For this review, use the dimensioned drawing (mm, ordinates from the lowest corner) and the shaded views. Give positions to 0.01 mm unless a question says otherwise; leave off trailing zeros. Loops run counter-clockwise (first coordinate to the right, second up) from the corner with the lowest first, then second, coordinate; pieces in that order, holes last. Notation, with made-up numbers: (-38.75, -27) -> (2.25, -27) arc R30 ccw to (2.25, 3) -> close; hole circle Ø4 at (32.5, 14). An arc over 180 degrees is marked (long way). Use a Markdown table: item, result. Add a question column.
1. Add section D-D (z = 43.5). State the section outline as (x, y) points.
2. Add section C-C (x = 2.2). Count the separate pieces of the cut face and the enclosed holes in it, and give its area (3 significant figures).
3. Add section B-B (z = 30). State the section outline as (x, y) points.
4. For pin 1 Ø4 at (y, z) = (79, 47.5) entering from -X, flat-tipped, find the tip position at first contact; note if it passes through.
5. To check wall thickness, follow line 1 (Y direction, x = 2.1, z = 35.5); line 2 (Y direction, x = 2.35, z = 44); line 3 (Z direction, x = 0.8, y = 74.5). State the ranges of each line that lie inside material, in increasing order.
6. Add section A-A (y = 44). State the section outline as (x, z) points, and give its area (3 significant figures).
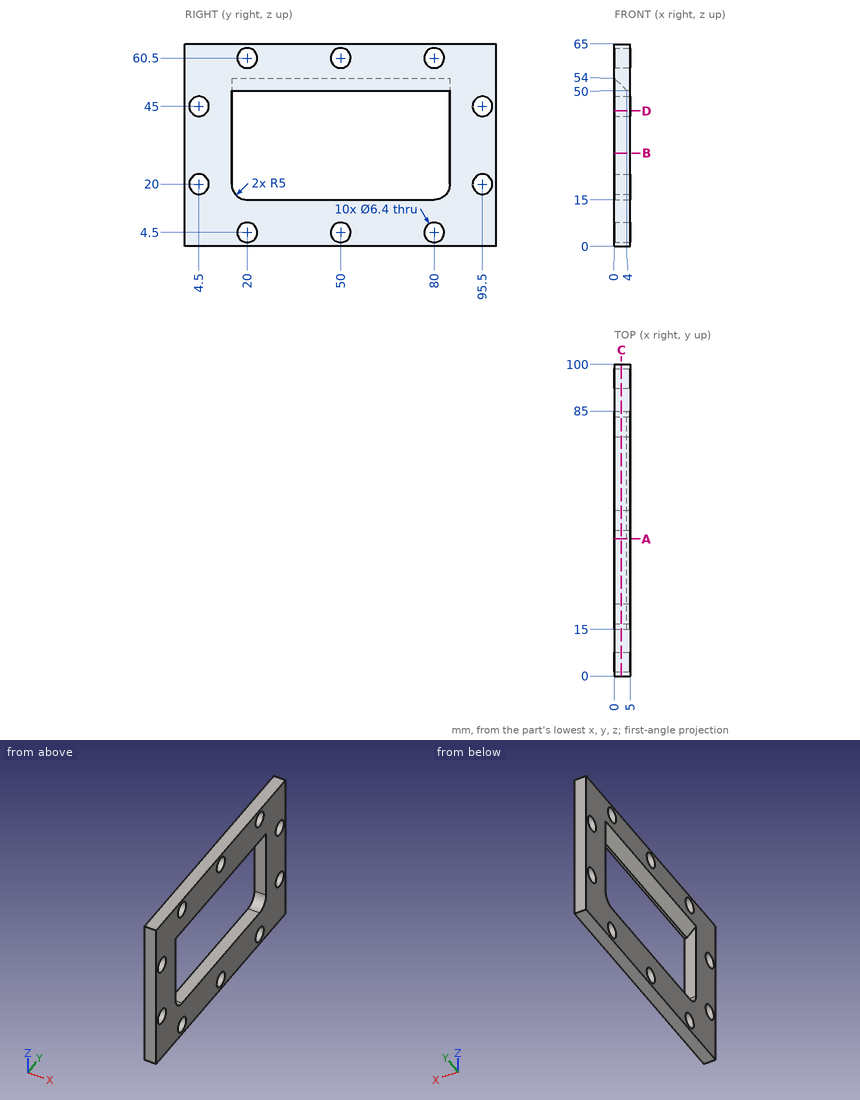
Taken from the geometry:
| question | item | result |
|---|---|---|
| 1 | outline | (0, 0) -> (5, 0) -> (5, 1.67) -> (0, 1.67) -> close; (0, 7.33) -> (5, 7.33) -> (5, 15) -> (0, 15) -> close; (0, 85) -> (5, 85) -> (5, 92.67) -> (0, 92.67) -> close; (0, 98.33) -> (5, 98.33) -> (5, 100) -> (0, 100) -> close |
| 2 | separate pieces | 1 |
| 2 | enclosed holes | 11 |
| 2 | area | 3,610 mm^2 |
| 3 | outline | (0, 0) -> (5, 0) -> (5, 15) -> (0, 15) -> close; (0, 85) -> (5, 85) -> (5, 100) -> (0, 100) -> close |
| 4 | pin 1 | passes through |
| 5 | line 1 | y = 0 to 15, 85 to 100 |
| 5 | line 2 | y = 0 to 1.46, 7.54 to 15, 85 to 92.46, 98.54 to 100 |
| 5 | line 3 | z = 0 to 15, 53.2 to 65 |
| 6 | outline | (0, 0) -> (5, 0) -> (5, 15) -> (0, 15) -> close; (0, 54) -> (4, 50) -> (5, 50) -> (5, 65) -> (0, 65) -> close |
| 6 | area | 142 mm^2 |
